from build123d import *

# Parameters (mm, degrees)
SKETCH_1_W          = 40
SKETCH_1_H          = 20
EXTRUDE_1_DEPTH     = 40
SKETCH_2_R          = 2
SKETCH_2_R_2        = 6
SKETCH_2_R_3        = 2.1
CUT_EXTRUDE_1_DEPTH = 46.82575695
CUT_EXTRUDE_2_DEPTH = 46.82575695
CUT_EXTRUDE_3_DEPTH = 46.82575695


with BuildPart() as part:
    # 스케치1 → 보스-돌출1 (new body)
    with BuildSketch(Plane.XY):
        Rectangle(SKETCH_1_W, SKETCH_1_H)
    extrude(amount=EXTRUDE_1_DEPTH)

    # 스케치2 → 컷-돌출1 (cut, through all)
    with BuildSketch(Plane.XY.offset(40)):
        with Locations((-17, 7)):
            Circle(SKETCH_2_R)
        with Locations((-17, -7)):
            Circle(SKETCH_2_R)
        with Locations((17, -7)):
            Circle(SKETCH_2_R)
        with Locations((17, 7)):
            Circle(SKETCH_2_R)
        Circle(SKETCH_2_R_2)
        with Locations((-10, 0)):
            Circle(SKETCH_2_R_3)
        with Locations(Location((10, 0, 0), (0, 0, 180))):
            Circle(SKETCH_2_R_3)
    extrude(amount=-CUT_EXTRUDE_1_DEPTH, mode=Mode.SUBTRACT)

    # 스케치3 → 컷-돌출2 (cut, through all)
    with BuildSketch(Plane(origin=(0, 0, 0), x_dir=(-1, 0, 0), z_dir=(0, 0, -1))):
        with BuildLine():
            Line((-20, 2.65), (-20, -2.65))
            Line((-20, -2.65), (-18.5, -2.65))
            Line((-18.5, -2.65), (-18.5, -4.15))
            Line((-18.5, -4.15), (-15.666698718, -4.15))
            ThreePointArc((-15.666698718, -4.15), (-14, 0), (-15.666698718, 4.15))
            Line((-15.666698718, 4.15), (-18.5, 4.15))
            Line((-18.5, 4.15), (-18.5, 2.65))
            Line((-18.5, 2.65), (-20, 2.65))
        make_face()
        with BuildLine():
            Line((-14.15, 8.5), (-14.15, 5.666698718))
            ThreePointArc((-14.15, 5.666698718), (-10, 4), (-5.85, 5.666698718))
            Line((-5.85, 5.666698718), (-5.85, 8.5))
            Line((-5.85, 8.5), (-7.35, 8.5))
            Line((-7.35, 8.5), (-7.35, 10))
            Line((-7.35, 10), (-12.65, 10))
            Line((-12.65, 10), (-12.65, 8.5))
            Line((-12.65, 8.5), (-14.15, 8.5))
        make_face()
        with BuildLine():
            Line((-12.65, -8.5), (-14.15, -8.5))
            Line((-14.15, -8.5), (-14.15, -5.666698718))
            ThreePointArc((-14.15, -5.666698718), (-10, -4), (-5.85, -5.666698718))
            Line((-5.85, -5.666698718), (-5.85, -8.5))
            Line((-5.85, -8.5), (-7.35, -8.5))
            Line((-7.35, -8.5), (-7.35, -10))
            Line((-7.35, -10), (-12.65, -10))
            Line((-12.65, -10), (-12.65, -8.5))
        make_face()
        with BuildLine():
            Line((14.15, -8.5), (14.15, -5.666698718))
            ThreePointArc((14.15, -5.666698718), (10, -4), (5.85, -5.666698718))
            Line((5.85, -5.666698718), (5.85, -8.5))
            Line((5.85, -8.5), (7.35, -8.5))
            Line((7.35, -8.5), (7.35, -10))
            Line((7.35, -10), (12.65, -10))
            Line((12.65, -10), (12.65, -8.5))
            Line((12.65, -8.5), (14.15, -8.5))
        make_face()
        with BuildLine():
            Line((12.65, 8.5), (14.15, 8.5))
            Line((14.15, 8.5), (14.15, 5.666698718))
            ThreePointArc((14.15, 5.666698718), (10, 4), (5.85, 5.666698718))
            Line((5.85, 5.666698718), (5.85, 8.5))
            Line((5.85, 8.5), (7.35, 8.5))
            Line((7.35, 8.5), (7.35, 10))
            Line((7.35, 10), (12.65, 10))
            Line((12.65, 10), (12.65, 8.5))
        make_face()
        with BuildLine():
            Line((18.5, -4.15), (15.666698718, -4.15))
            ThreePointArc((15.666698718, -4.15), (14, 0), (15.666698718, 4.15))
            Line((15.666698718, 4.15), (18.5, 4.15))
            Line((18.5, 4.15), (18.5, 2.65))
            Line((18.5, 2.65), (20, 2.65))
            Line((20, 2.65), (20, -2.65))
            Line((20, -2.65), (18.5, -2.65))
            Line((18.5, -2.65), (18.5, -4.15))
        make_face()
    extrude(amount=-CUT_EXTRUDE_2_DEPTH, mode=Mode.SUBTRACT)

    # 스케치4 → 컷-돌출3 (cut, through all)
    with BuildSketch(Plane(origin=(0, 0, 0), x_dir=(-1, 0, 0), z_dir=(0, 0, -1))):
        with BuildLine():
            Line((-3.35, 8.5), (3.35, 8.5))
            ThreePointArc((3.35, 8.5), (4.057106781, 8.207106781), (4.35, 7.5))
            Line((4.35, 7.5), (4.35, -7.5))
            ThreePointArc((4.35, -7.5), (4.057106781, -8.207106781), (3.35, -8.5))
            Line((3.35, -8.5), (-3.35, -8.5))
            ThreePointArc((-3.35, -8.5), (-4.057106781, -8.207106781), (-4.35, -7.5))
            Line((-4.35, -7.5), (-4.35, 7.5))
            ThreePointArc((-4.35, 7.5), (-4.057106781, 8.207106781), (-3.35, 8.5))
        make_face()
    extrude(amount=-CUT_EXTRUDE_3_DEPTH, mode=Mode.SUBTRACT)


solid = part.part
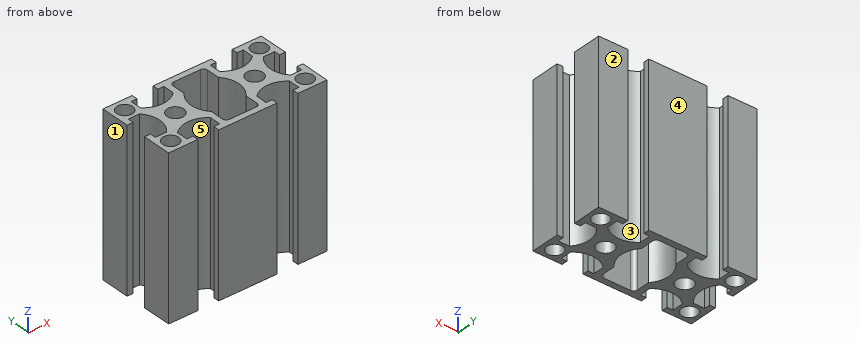
Geometry check sheet. Reference: the model listing, model coordinates, mm. Face numbers are marked on the shaded views. A direction names the side the tool comes from. Give positions to 0.01 mm unless a question says otherwise; leave off trailing zeros. Loops run counter-clockwise (first coordinate to the right, second up) from the corner with the lowest first, then second, coordinate; pieces in that order, holes last.
(1) Section check D-D on x = -17. Record the cut outline in (y, z), then the cut area to 3 significant figures.
From the geometry:
outline: (-10, 0) - (-9, 0) - (-9, 40) - (-10, 40) - close; (-5, 0) - (-4.15, 0) - (-4.15, 40) - (-5, 40) - close; (4.15, 0) - (5, 0) - (5, 40) - (4.15, 40) - close; (9, 0) - (10, 0) - (10, 40) - (9, 40) - close
area: 148 mm2
(2) Depth check by flat-ended pin: pin 1 Ø1 at (y, z) = (-2, 35.5) entering from +X; pin 2 Ø2 at (x, z) = (-9.5, 28) entering from -Y. Enter the tip coordinate at first touch or a pass-through.
From the geometry:
pin 1: stops at x = 14.55
pin 2: stops at y = -4.19
(3) Release check for a two-part mould opening along X. For the marked faces 1, 2 and 3 record: released by +X, released by -X, zero draft, split by the parting line, or undercut.
From the geometry:
face 1: released by -X
face 2: zero draft
face 3: undercut
(4) Section check C-C on y = -3.25. Record the cut outline in (x, z), then the cut area to 3 significant figures.
From the geometry:
outline: (-20, 0) - (-18.5, 0) - (-18.5, 40) - (-20, 40) - close; (-14.96, 0) - (-5.04, 0) - (-5.04, 40) - (-14.96, 40) - close; (5.04, 0) - (14.96, 0) - (14.96, 40) - (5.04, 40) - close; (18.5, 0) - (20, 0) - (20, 40) - (18.5, 40) - close
area: 913 mm2
(5) Set-up check for the marked faces 4 and 5: record each of +Z, -Z, +X, -X, +Y, -Y from which the full face is reachable in a straight line by a thin tool's end or side.
From the geometry:
face 4: +Z, -Z, +X, -X, +Y
face 5: +Z, -Z
(6) Section check B-B on y = 7. Record the cut outline in (x, z), then the cut area to 3 significant figures.
From the geometry:
outline: (-20, 0) - (-19, 0) - (-19, 40) - (-20, 40) - close; (-15, 0) - (-14.15, 0) - (-14.15, 40) - (-15, 40) - close; (-5.85, 0) - (-4.35, 0) - (-4.35, 40) - (-5.85, 40) - close; (4.35, 0) - (5.85, 0) - (5.85, 40) - (4.35, 40) - close; (14.15, 0) - (15, 0) - (15, 40) - (14.15, 40) - close; (19, 0) - (20, 0) - (20, 40) - (19, 40) - close
area: 268 mm2
(7) Thickness scan on L1, parallel to Y at x = 17, z = 27; L2, parallel to Y at x = 6.5, z = 29; L3, parallel to X at y = 4.5, z = 16.5. Record the ranges inside material, lowest first.
From the geometry:
L1: y = -10 to -9, -5 to -4.15, 4.15 to 5, 9 to 10
L2: y = -10 to -8.5, -5.13 to 5.13, 8.5 to 10
L3: x = -20 to -12.4, -7.6 to -4.35, 4.35 to 7.6, 12.4 to 20
(8) Section check A-A on x = 2. Record the cut outline in (y, z).
From the geometry:
outline: (-10, 0) - (-8.5, 0) - (-8.5, 40) - (-10, 40) - close; (8.5, 0) - (10, 0) - (10, 40) - (8.5, 40) - close
